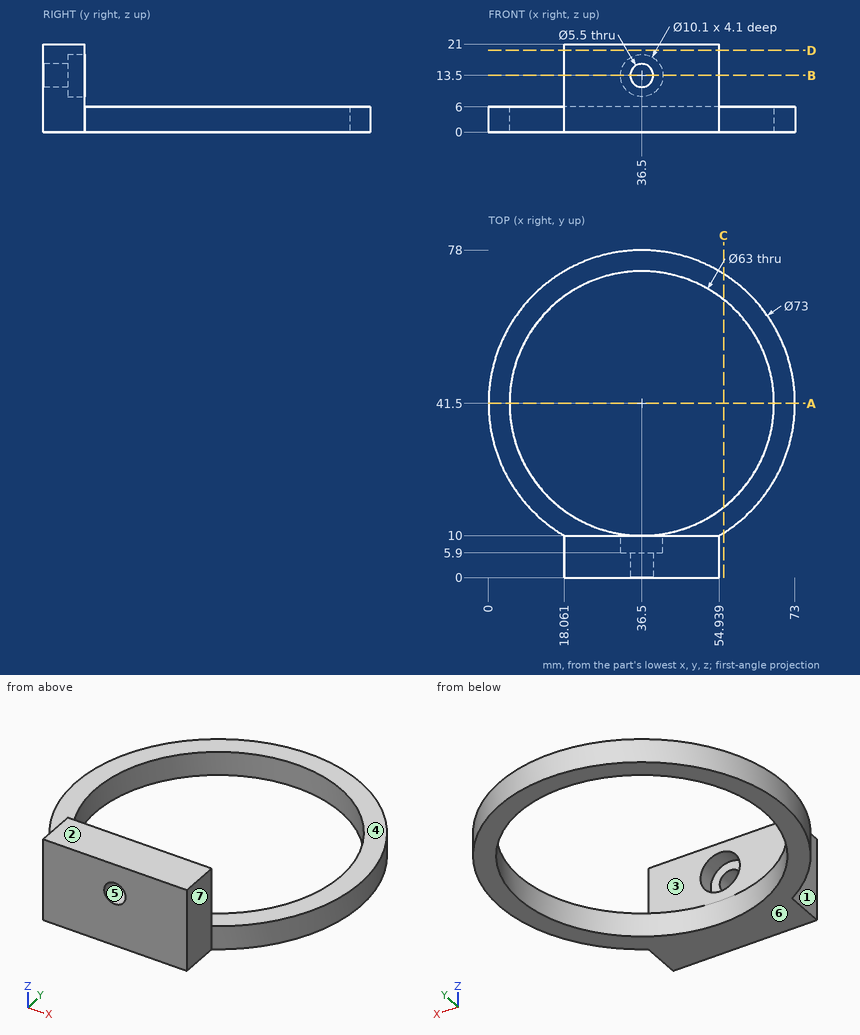
Check sheet for the drawn part. Datum: minimum x, y, z corner. Units: mm. A direction names the side the tool comes from. Give positions to 0.01 mm unless a question says otherwise; leave off trailing zeros. Loops run counter-clockwise (first coordinate to the right, second up) from the corner with the lowest first, then second, coordinate; pieces in that order, holes last.
1) Sectioned sample at B-B, the plane z = 13.5. Enter the section's corners in (x, y).
2) Sectioned sample at D-D, the plane z = 19.5. Enter the section's corners in (x, y).
3) Depth check by flat-ended pin: pin 1 Ø10 at (x, y) = (52, 15.5) entering from -Z; pin 2 Ø8 at (y, z) = (4, 10.5) entering from -X; pin 3 Ø3 at (y, z) = (3, 10) entering from +X; pin 4 Ø8 at (x, z) = (39.5, 14.5) entering from +Y. Enter the tip coordinate at first touch or a pass-through.
4) Set-up check for the marked faces 1, 2 and 3: record each of +Z, -Z, +X, -X, +Y, -Y from which the full face is reachable in a straight line by a thin tool's end or side.
5) Thickness scan on line 1 along X through (y, z) = (41.5, 3.5); line 2 along Z through (x, y) = (36.5, 7.2); line 3 along Y through (x, z) = (34.5, 11.5). Record the ranges inside material, lowest first.
6) Draft check along Z on the marked faces 4, 5, 6 and 7. Enter one of: pulls with the +Z half, pulls with the -Z half, needs draft (parallel to the pull), parting line crosses it, or undercut.
7) Sectioned sample at C-C, the plane x = 56. Enter the section's corners in (y, z).
8) Sectioned sample at A-A, the plane y = 41.5. Enter the section's corners in (x, z), then the cut area to 3 significant figures.
Answers:
1. outline: (18.06, 0) - (33.75, 0) - (33.75, 5.9) - (31.45, 5.9) - (31.45, 10) - (18.06, 10) - close; (39.25, 0) - (54.94, 0) - (54.94, 10) - (41.55, 10) - (41.55, 5.9) - (39.25, 5.9) - close
2. outline: (18.06, 0) - (54.94, 0) - (54.94, 10) - (18.06, 10) - close
3. pin 1: stops at z = 0
3. pin 2: stops at x = 18.06
3. pin 3: stops at x = 54.94
3. pin 4: stops at y = 10
4. face 1: +Z, -Z, -X, -Y
4. face 2: +Z, +X, -X, +Y, -Y
4. face 3: +Z, +X, -X, +Y
5. line 1: x = 0 to 5, 68 to 73
5. line 2: z = 0 to 8.45, 18.55 to 21
5. line 3: y = 0 to 5.9
6. face 4: pulls with the +Z half
6. face 5: undercut
6. face 6: pulls with the -Z half
6. face 7: needs draft
7. outline: (10.65, 0) - (16.76, 0) - (16.76, 6) - (10.65, 6) - close; (66.24, 0) - (72.35, 0) - (72.35, 6) - (66.24, 6) - close
8. outline: (0, 0) - (5, 0) - (5, 6) - (0, 6) - close; (68, 0) - (73, 0) - (73, 6) - (68, 6) - close
8. area: 60.0 mm2
